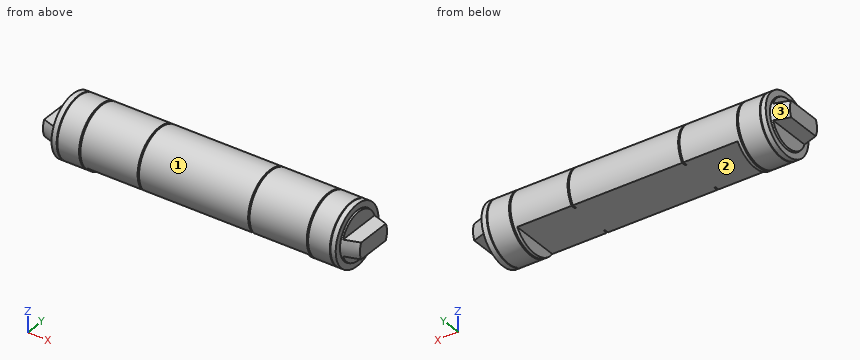
```python
from build123d import *

# Parameters (mm, degrees)
CUT_EXTRUDE_1_DEPTH      = 167.845737135
CUT_EXTRUDE_1_DEPTH_BACK = 167.845737135
SKETCH_2_W               = 128
SKETCH_2_H               = 19.899130277
SKETCH_3_R               = 14
EXTRUDE_1_DEPTH          = 9.5
EXTRUDE_1_TAPER          = 17
SKETCH_4_W               = 17.504538799
SKETCH_4_H               = 43.451593783
CUT_EXTRUDE_2_DEPTH      = 8.5
SKETCH_5_R               = 14
EXTRUDE_2_DEPTH          = 9.5
EXTRUDE_2_TAPER          = 17
SKETCH_6_W               = 11.469588706
SKETCH_6_H               = 34.444631615
CUT_EXTRUDE_3_DEPTH      = 8.5


with BuildPart() as part:
    # Sketch 1 → Revolve 1 (revolve)
    with BuildSketch(Plane(origin=(0, 0, 0), x_dir=(1, 0, 0), z_dir=(0, 1, 0)), mode=Mode.PRIVATE) as revolve_1_sk:
        Polygon((0, 0), (0, 17.5), (3, 17.5), (3, 15.5), (3.4, 15.5), (3.4, 17.5), (16, 17.5), (16, 15.5), (16.8, 15.5), (16.8, 17.5), (50, 17.5), (50, 15.5), (50.8, 15.5), (50.8, 17.5), (114.2, 17.5), (114.2, 15.5), (115, 15.5), (115, 17.5), (148.2, 17.5), (148.2, 15.5), (149, 15.5), (149, 17.5), (161.6, 17.5), (161.6, 15.5), (162, 15.5), (162, 17.5), (165, 17.5), (165, 0), align=None)
    revolve(revolve_1_sk.sketch.rotate(Axis((0, 0, 0), (1, 0, 0)), 180), axis=Axis((0, 0, 0), (1, 0, 0)))

    # Sketch 2 → Cut-Extrude 1 (cut, two sides: drawn at the far end of the back side and taken through both)
    with BuildSketch(Plane(origin=(0, 0, 0), x_dir=(1, 0, 0), z_dir=(0, 1, 0)).offset(-CUT_EXTRUDE_1_DEPTH_BACK)):
        with Locations((82.5, 19.949565138)):
            Rectangle(SKETCH_2_W, SKETCH_2_H)
    extrude(amount=CUT_EXTRUDE_1_DEPTH + CUT_EXTRUDE_1_DEPTH_BACK, mode=Mode.SUBTRACT)

    # Sketch 3 → Extrude 1 (add)
    with BuildSketch(Plane.ZY):
        Circle(SKETCH_3_R)
    extrude(amount=EXTRUDE_1_DEPTH, taper=EXTRUDE_1_TAPER)

    # Sketch 4 → Cut-Extrude 2 (cut)
    with BuildSketch(Plane.ZY.offset(9.5)):
        with Locations((-13.5022694, 0.56408101)):
            Rectangle(SKETCH_4_W, SKETCH_4_H)
        with Locations((13.5022694, 0.56408101)):
            Rectangle(SKETCH_4_W, SKETCH_4_H)
    extrude(amount=-CUT_EXTRUDE_2_DEPTH, mode=Mode.SUBTRACT)

    # Sketch 5 → Extrude 2 (add)
    with BuildSketch(Plane(origin=(165, 0, 0), x_dir=(0, 0, -1), z_dir=(1, 0, 0))):
        Circle(SKETCH_5_R)
    extrude(amount=EXTRUDE_2_DEPTH, taper=EXTRUDE_2_TAPER)

    # Sketch 6 → Cut-Extrude 3 (cut)
    with BuildSketch(Plane(origin=(174.5, 0, 0), x_dir=(0, 0, -1), z_dir=(1, 0, 0))):
        with Locations((10.484794353, 0.773198928)):
            Rectangle(SKETCH_6_W, SKETCH_6_H)
        with Locations((-10.484794353, 0.773198928)):
            Rectangle(SKETCH_6_W, SKETCH_6_H)
    extrude(amount=-CUT_EXTRUDE_3_DEPTH, mode=Mode.SUBTRACT)


solid = part.part
```
The listing builds one solid part. Answer for the finished solid, in the listing's coordinates (mm). Face numbers are marked on the shaded views. Round coordinates to 2 decimals unless told otherwise and drop trailing zeros. Write each loop counter-clockwise with the first axis right and the second up, starting at its lowest first coordinate (ties: lowest second). Pieces come first, ordered by that corner, then holes. Notation, with made-up numbers: (40, 29.5) -> (98, 29.5) arc R11 ccw to (98, 40.5) -> close; hole circle Ø10 at (2, 0.25). An arc over 180 degrees is marked (long way). Answer as a JSON object with one key per item and string values. Group by question number.
Q1. Straight lines are drawn through the part: line 1 along X through (y, z) = (-8, -13.5); line 2 along X through (y, z) = (-3, -11); line 3 along X through (y, z) = (-1, 11). For each, find the intervals that lie inside material, in ascending order.
Q2. Each of these flat-tipped pins is pushed along its axis until it touches: pin 1 Ø8.5 at (y, z) = (7, -13.5) entering from +X; pin 2 Ø1.5 at (x, z) = (111.5, -1.5) entering from -Y; pin 3 Ø2.5 at (y, z) = (7, -14) entering from -X. Where does it stop, or does it pass through?
Q3. Section A-A (x = 109) is taken. Write down the section's boundary in (y, z).
Q4. Determine the mould class of the marked faces 1, 2 and 3 for opening direction X: pulls with the +X half, pulls with the -X half, needs draft (parallel to the pull), parting line crosses it, or undercut.
Check values:
{
 "1": {"line 1": "0 to 3, 3.4 to 16, 16.8 to 18.5, 146.5 to 148.2, 149 to 161.6, 162 to 165", "line 2": "-1 to 18.5, 146.5 to 166", "line 3": "-1 to 166"},
 "2": {"pin 1": "x = 166", "pin 2": "y = -17.48", "pin 3": "x = 0"},
 "3": {"outline": "(-14.36, -10) -> (14.36, -10) arc R17.5 ccw (long way) to start"},
 "4": {"face 1": "needs draft", "face 2": "undercut", "face 3": "pulls with the -X half"}
}
